Check sheet for the drawn part. Datum: minimum x, y, z corner. Units: mm. A direction names the side the tool comes from. Give positions to 0.01 mm unless a question says otherwise; leave off trailing zeros. Write each loop counter-clockwise with the first axis right and the second up, starting at its lowest first coordinate (ties: lowest second). Pieces come first, ordered by that corner, then holes.
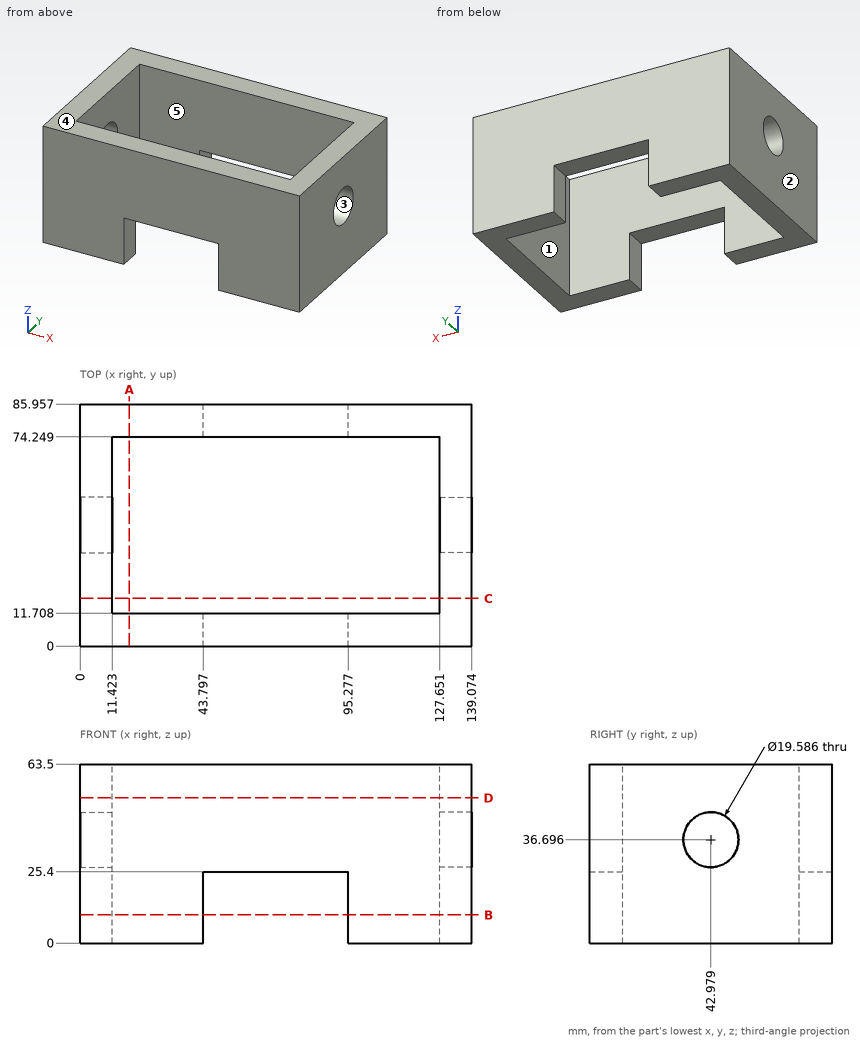
1) Scan lines: L1, parallel to X at y = 8, z = 3; L2, parallel to X at y = 69.5, z = 27; L3, parallel to Y at x = 74.5, z = 44.5. Record each from-to range of solid material in increasing order.
2) Draft check along Z on the marked faces 3, 4 and 5. Enter one of: +Z half, -Z half, draft (parallel to the pull), parting line (faces both ways), or undercut.
3) Sectioned sample at A-A on x = 17.5. Record the boundary of the cut face in (y, z).
4) Sectioned sample at B-B on z = 10. Record the boundary of the cut face in (x, y).
5) Access from +Z, -Z, +X, -X, +Y, -Y to the whole of each face (thin tool, end or side, straight path). Record for the marked faces 1 and 2.
6) Sectioned sample at C-C on y = 17. Record the boundary of the cut face in (x, z), then the cut area to 3 significant figures.
7) Gauge pin test, flat ends, axial feed: pin 1 (9.5 mm diameter, centred on x = 58, y = 5, fed in from -Z); pin 2 (19 mm diameter, centred on x = 86, z = 17, fed in from -Y). Record the tip position at first contact, or that the pin passes through.
8) Sectioned sample at D-D on z = 51.5. Record the boundary of the cut face in (x, y).
Answers below:
1. L1: x = 0 to 43.8, 95.28 to 139.07
1. L2: x = 0 to 11.42, 127.65 to 139.07
1. L3: y = 0 to 11.71, 74.25 to 85.96
2. face 3: undercut
2. face 4: +Z half
2. face 5: draft
3. outline: (0, 0) - (11.71, 0) - (11.71, 63.5) - (0, 63.5) - close; (74.25, 0) - (85.96, 0) - (85.96, 63.5) - (74.25, 63.5) - close
4. outline: (0, 0) - (43.8, 0) - (43.8, 11.71) - (11.42, 11.71) - (11.42, 74.25) - (43.8, 74.25) - (43.8, 85.96) - (0, 85.96) - close; (95.28, 0) - (139.07, 0) - (139.07, 85.96) - (95.28, 85.96) - (95.28, 74.25) - (127.65, 74.25) - (127.65, 11.71) - (95.28, 11.71) - close
5. face 1: +Z, -Z
5. face 2: +Z, -Z, -X, +Y, -Y
6. outline: (0, 0) - (11.42, 0) - (11.42, 63.5) - (0, 63.5) - close; (127.65, 0) - (139.07, 0) - (139.07, 63.5) - (127.65, 63.5) - close
6. area: 1,450 mm2
7. pin 1: stops at z = 25.4
7. pin 2: stops at y = 0
8. outline: (0, 0) - (139.07, 0) - (139.07, 85.96) - (0, 85.96) - close; hole (11.42, 11.71) - (127.65, 11.71) - (127.65, 74.25) - (11.42, 74.25) - close
